For this review, take the finished solid that the model builds, in its own axes (mm). A direction names the side the tool comes from. Coordinates: 2 decimals unless noted, no trailing zeros. Write each loop counter-clockwise with the first axis right and the second up, starting at its lowest first coordinate (ties: lowest second). Pieces come first, ordered by that corner, then holes. Notation, with made-up numbers: M -17,51 L 8,51 A13 cw 8,58 Z; hole C 19.25,63 d9. An arc over 180 degrees is marked long. Return JSON: item names as keys, results as strings.
```python
from build123d import *

# Parameters (mm, degrees)
SKETCH1_W           = 60
SKETCH1_H           = 45
BOSS_EXTRUDE1_DEPTH = 10
SKETCH2_W           = 25.78
SKETCH2_H           = 34.5
CUT_EXTRUDE1_DEPTH  = 5
CUT_EXTRUDE2_REACH  = 48.312
SKETCH3_R           = 1.15
SKETCH4_W           = 14.64
SKETCH4_H           = 23.95
CUT_EXTRUDE3_DEPTH  = 5
CUT_EXTRUDE4_REACH  = 48.312
SKETCH5_R           = 1.015
FILLET1_R           = 5
FILLET2_R           = 5
FILLET3_R           = 5
FILLET4_R           = 3
CUT_EXTRUDE5_REACH  = 49.115
SKETCH6_R           = 1.7


with BuildPart() as part:
    # Sketch1 → Boss-Extrude1 (new body)
    with BuildSketch(Plane(origin=(0, 0, 0), x_dir=(1, 0, 0), z_dir=(0, 1, 0))):
        with Locations((-9.130434783, -1.760869565)):
            Rectangle(SKETCH1_W, SKETCH1_H)
    extrude(amount=BOSS_EXTRUDE1_DEPTH)

    # Sketch2 → Cut-Extrude1 (cut)
    with BuildSketch(Plane(origin=(0, 10, 0), x_dir=(1, 0, 0), z_dir=(0, 1, 0))):
        with Locations((-26.240434783, -7.010869565)):
            Rectangle(SKETCH2_W, SKETCH2_H)
    extrude(amount=-CUT_EXTRUDE1_DEPTH, mode=Mode.SUBTRACT)

    # Sketch3 → Cut-Extrude2 (cut, up to next)
    with BuildSketch(Plane(origin=(0, 5, 0), x_dir=(1, 0, 0), z_dir=(0, 1, 0)), mode=Mode.PRIVATE) as cut_extrude2_sk1:
        with Locations(Location((-36.060434783, 6.939130435, 0), (0, 0, 270))):
            Circle(SKETCH3_R)
    cut_extrude2_tool1 = extrude(cut_extrude2_sk1.sketch, amount=-CUT_EXTRUDE2_REACH, mode=Mode.PRIVATE) & part.part
    # Sketch3 → Cut-Extrude2 (cut, up to next)
    with BuildSketch(Plane(origin=(0, 5, 0), x_dir=(1, 0, 0), z_dir=(0, 1, 0)), mode=Mode.PRIVATE) as cut_extrude2_sk2:
        with Locations(Location((-16.640434783, -21.370869565, 0), (0, 0, 270))):
            Circle(SKETCH3_R)
    cut_extrude2_tool2 = extrude(cut_extrude2_sk2.sketch, amount=-CUT_EXTRUDE2_REACH, mode=Mode.PRIVATE) & part.part
    add(cut_extrude2_tool1.solids().sort_by_distance((-36.060435, 5, -6.93913))[0], mode=Mode.SUBTRACT)
    add(cut_extrude2_tool2.solids().sort_by_distance((-16.640435, 5, 21.37087))[0], mode=Mode.SUBTRACT)

    # Sketch4 → Cut-Extrude3 (cut)
    with BuildSketch(Plane(origin=(0, 10, 0), x_dir=(1, 0, 0), z_dir=(0, 1, 0))):
        with Locations((-1.030434783, -12.285869565)):
            Rectangle(SKETCH4_W, SKETCH4_H)
    extrude(amount=-CUT_EXTRUDE3_DEPTH, mode=Mode.SUBTRACT)

    # Sketch5 → Cut-Extrude4 (cut, up to next)
    with BuildSketch(Plane(origin=(0, 5, 0), x_dir=(1, 0, 0), z_dir=(0, 1, 0)), mode=Mode.PRIVATE) as cut_extrude4_sk1:
        with Locations(Location((4.244565217, -2.330869565, 0), (0, 0, 270))):
            Circle(SKETCH5_R)
    cut_extrude4_tool1 = extrude(cut_extrude4_sk1.sketch, amount=-CUT_EXTRUDE4_REACH, mode=Mode.PRIVATE) & part.part
    # Sketch5 → Cut-Extrude4 (cut, up to next)
    with BuildSketch(Plane(origin=(0, 5, 0), x_dir=(1, 0, 0), z_dir=(0, 1, 0)), mode=Mode.PRIVATE) as cut_extrude4_sk2:
        with Locations(Location((4.239565217, -22.245869565, 0), (0, 0, 270))):
            Circle(SKETCH5_R)
    cut_extrude4_tool2 = extrude(cut_extrude4_sk2.sketch, amount=-CUT_EXTRUDE4_REACH, mode=Mode.PRIVATE) & part.part
    add(cut_extrude4_tool1.solids().sort_by_distance((4.244565, 5, 2.33087))[0], mode=Mode.SUBTRACT)
    add(cut_extrude4_tool2.solids().sort_by_distance((4.239565, 5, 22.24587))[0], mode=Mode.SUBTRACT)

    # Fillet1
    fillet1_edges = [part.edges().sort_by_distance(p)[0] for p in [
        (-39.130434783, 5, -20.739130435),
    ]]
    fillet(fillet1_edges, radius=FILLET1_R)

    # Fillet2
    fillet2_edges = [part.edges().sort_by_distance(p)[0] for p in [
        (20.869565217, 5, -20.739130435),
    ]]
    fillet(fillet2_edges, radius=FILLET2_R)

    # Fillet3
    fillet3_edges = [part.edges().sort_by_distance(p)[0] for p in [
        (20.869565217, 5, 24.260869565),
    ]]
    fillet(fillet3_edges, radius=FILLET3_R)

    # Fillet4
    fillet4_edges = [part.edges().sort_by_distance(p)[0] for p in [
        (-10.850434783, 10, 24.260869565),
        (11.079565217, 10, 24.260869565),
        (-39.130434783, 10, -12.989130435),
        (-37.665968689, 10, -19.274664341),
        (-9.130434783, 10, -20.739130435),
        (19.405099123, 10, -19.274664341),
        (20.869565217, 10, 1.760869565),
        (19.405099123, 10, 22.796403471),
    ]]
    fillet(fillet4_edges, radius=FILLET4_R)

    # Sketch6 → Cut-Extrude5 (cut, up to next)
    with BuildSketch(Plane(origin=(0, 10, 0), x_dir=(1, 0, 0), z_dir=(0, 1, 0)), mode=Mode.PRIVATE) as cut_extrude5_sk1:
        with Locations(Location((-33.790434783, 15.395190435, 0), (0, 0, 270))):
            Circle(SKETCH6_R)
    cut_extrude5_tool1 = extrude(cut_extrude5_sk1.sketch, amount=-CUT_EXTRUDE5_REACH, mode=Mode.PRIVATE) & part.part
    # Sketch6 → Cut-Extrude5 (cut, up to next)
    with BuildSketch(Plane(origin=(0, 10, 0), x_dir=(1, 0, 0), z_dir=(0, 1, 0)), mode=Mode.PRIVATE) as cut_extrude5_sk2:
        with Locations(Location((15.529565217, 15.399130435, 0), (0, 0, 270))):
            Circle(SKETCH6_R)
    cut_extrude5_tool2 = extrude(cut_extrude5_sk2.sketch, amount=-CUT_EXTRUDE5_REACH, mode=Mode.PRIVATE) & part.part
    # Sketch6 → Cut-Extrude5 (cut, up to next)
    with BuildSketch(Plane(origin=(0, 10, 0), x_dir=(1, 0, 0), z_dir=(0, 1, 0)), mode=Mode.PRIVATE) as cut_extrude5_sk3:
        with Locations(Location((15.529565217, -18.920869565, 0), (0, 0, 270))):
            Circle(SKETCH6_R)
    cut_extrude5_tool3 = extrude(cut_extrude5_sk3.sketch, amount=-CUT_EXTRUDE5_REACH, mode=Mode.PRIVATE) & part.part
    add(cut_extrude5_tool1.solids().sort_by_distance((-33.790435, 10, -15.39519))[0], mode=Mode.SUBTRACT)
    add(cut_extrude5_tool2.solids().sort_by_distance((15.529565, 10, -15.39913))[0], mode=Mode.SUBTRACT)
    add(cut_extrude5_tool3.solids().sort_by_distance((15.529565, 10, 18.92087))[0], mode=Mode.SUBTRACT)


solid = part.part
```
1. For faces 5 (the face through (-26, 5, 7)), 6 (the face through (-1, 5, 12)), 7 (the face through (-10.815, 9.098, 23.405)), list the 3-axis set-ups (+Z, -Z, +X, -X, +Y, -Y) from which the entire face can be reached by the end or side of a thin tool; tool diameter is ignored.
Checks:
{"face 5": "+Z, -X, +Y", "face 6": "+Z, +Y", "face 7": "+Z, +X, -X, +Y"}
2. Draft analysis for pull direction Z (two halves, no side actions). For faces 1 (the face through (6.29, 8, 12)), 2 (the face through (3.62, 2.54, 21.44)), 3 (the face through (-12, 3, 24.261)), 4 (the face through (19.37, 3.55, -19.31)), state which applies: +Z half, -Z half, draft (parallel to the pull), parting line (faces both ways), or undercut.
Checks:
{"face 1": "draft", "face 2": "undercut", "face 3": "+Z half", "face 4": "-Z half"}
3. Clearance check with flat-ended pins moving along their axes: pin 1 Ø4.5 at (x, z) = (1, 8.5) entering from +Y; pin 2 Ø5 at (x, y) = (1, 8.5) entering from +Z; pin 3 Ø1.8 at (x, z) = (-36.06, -6.94) entering from +Y; pin 4 Ø1.5 at (x, y) = (10, 8) entering from +Z. State where each tip first meets the part, or that it passes through.
Checks:
{"pin 1": "y = 5", "pin 2": "z = 0.31", "pin 3": "through", "pin 4": "z = 24.25"}
4. We need section C-C (x = -18.5). State the section outline as (y, z) points, plus the area to 3 significant figures.
Checks:
{"outline": "M 0,-20.74 L 7,-20.74 A3 ccw 10,-17.74 L 10,-10.24 L 5,-10.24 L 5,24.26 L 0,24.26 Z", "area": "276 mm2"}
5. We need section A-A (z = -2). State the section outline as (x, y) points.
Checks:
{"outline": "M -39.13,0 L 20.87,0 L 20.87,7 A3 ccw 17.87,10 L -13.35,10 L -13.35,5 L -39.13,5 Z"}
6. We need section D-D (z = 18). State the section outline as (x, y) points.
Checks:
{"outline": "M -39.13,0 L 14.1,0 L 14.1,10 L 6.29,10 L 6.29,5 L -8.35,5 L -8.35,10 L -13.35,10 L -13.35,5 L -39.13,5 Z; M 16.96,0 L 20.87,0 L 20.87,7 A3 ccw 17.87,10 L 16.96,10 Z"}
7. We need section B-B (y = 4.25). State the section outline as (x, z) points (3 decimals).
Checks:
{"outline": "M -39.13,-15.739 A5 ccw -34.13,-20.739 L 15.87,-20.739 A5 ccw 20.87,-15.739 L 20.87,19.261 A5 ccw 15.87,24.261 L -39.13,24.261 Z; hole C -36.06,-6.939 d2.3; hole C -33.79,-15.395 d3.4; hole C -16.64,21.371 d2.3; hole C 4.24,22.246 d2.03; hole C 4.245,2.331 d2.03; hole C 15.53,-15.399 d3.4; hole C 15.53,18.921 d3.4"}
8. Wall thickness on L1, parallel to X at y = 7.25, z = 19; L2, parallel to Z at x = -34, y = 2.75; L3, parallel to Z at x = 15, y = 8: over which ranges is each line inside the solid? List them lowest first. Write a range as from..to.
Checks:
{"L1": "-13.35..-8.35, 6.29..13.83, 17.23..20.86", "L2": "-20.74..-17.08, -13.71..24.26", "L3": "-20.57..-17.01, -13.78..17.31, 20.54..24.09"}
